Could you check a few things on this model? Use its own coordinates, in mm. A direction names the side the tool comes from. Give positions to 0.01 mm unless a question says otherwise; leave off trailing zeros. Write each loop counter-clockwise with the first axis right and the second up, starting at its lowest first coordinate (ties: lowest second). Pieces come first, ordered by that corner, then holes. Notation, with made-up numbers: M 49,-23 L 63,-23 A26 ccw 63,12 Z; hole C 78,-2.5 d1. An arc over 180 degrees is marked long. One line per item, written item: value.
```python
from build123d import *

# Parameters (mm, degrees)
BOSS_EXTRUDE1_DEPTH      = 7
BOSS_EXTRUDE2_DEPTH      = 1
SKETCH3_W                = 6.66403437
SKETCH3_H                = 33.73555596
CUT_EXTRUDE1_DEPTH       = 29.374724668
BOSS_EXTRUDE3_DEPTH      = 3.3
CUT_EXTRUDE2_DEPTH       = 3.7
SKETCH6_W                = 4
SKETCH6_H                = 16.6
CUT_EXTRUDE3_DEPTH       = 2.5
BOSS_EXTRUDE4_REACH      = 45.389
BOSS_EXTRUDE4_END_RADIUS = 19.25
SKETCH7_R                = 1.5


with BuildPart() as part:
    # Sketch1 → Boss-Extrude1 (new body)
    with BuildSketch(Plane(origin=(0, 0, 0), x_dir=(1, 0, 0), z_dir=(0, 1, 0))):
        with BuildLine():
            Line((-16, -10.703387314), (-16, 10.703387314))
            ThreePointArc((-16, 10.703387314), (19.25, 0), (-16, -10.703387314))
        make_face()
        with BuildLine():
            Line((-15, -10.395311443), (-15, 10.395311443))
            ThreePointArc((-15, 10.395311443), (18.25, 0), (-15, -10.395311443))
        make_face(mode=Mode.SUBTRACT)
    extrude(amount=BOSS_EXTRUDE1_DEPTH)

    # Sketch2 → Boss-Extrude2 (add)
    with BuildSketch(Plane.XZ):
        with BuildLine():
            Line((-16, 10.703387314), (-16, -10.703387314))
            ThreePointArc((-16, -10.703387314), (19.25, 0), (-16, 10.703387314))
        make_face()
    extrude(amount=BOSS_EXTRUDE2_DEPTH)

    # Sketch3 → Cut-Extrude1 (cut, through all)
    with BuildSketch(Plane(origin=(0, 7, 0), x_dir=(1, 0, 0), z_dir=(0, 1, 0))):
        with Locations((-18.332017185, -0.479198238)):
            Rectangle(SKETCH3_W, SKETCH3_H)
    extrude(amount=-CUT_EXTRUDE1_DEPTH, mode=Mode.SUBTRACT)

    # Sketch4 → Boss-Extrude3 (add)
    with BuildSketch(Plane(origin=(0, 0, 0), x_dir=(1, 0, 0), z_dir=(0, 1, 0))):
        Polygon((-15, 12.064928512), (-15, -12.064928512), (-13, -12.808688457), (-13, 12.808688457), align=None)
    extrude(amount=BOSS_EXTRUDE3_DEPTH)

    # Sketch5 → Cut-Extrude2 (cut)
    with BuildSketch(Plane(origin=(0, 7, 0), x_dir=(1, 0, 0), z_dir=(0, 1, 0))):
        Polygon((0, 0), (-15, -12.064928512), (-15, 12.064928512), align=None)
    extrude(amount=-CUT_EXTRUDE2_DEPTH, mode=Mode.SUBTRACT)

    # Sketch6 → Cut-Extrude3 (cut)
    with BuildSketch(Plane(origin=(0, 3.3, 0), x_dir=(1, 0, 0), z_dir=(0, 1, 0))):
        with Locations((-15, 0)):
            Rectangle(SKETCH6_W, SKETCH6_H)
    extrude(amount=-CUT_EXTRUDE3_DEPTH, mode=Mode.SUBTRACT)

    # Boss-Extrude4: up to this cylinder (the profile starts outside it)
    boss_extrude4_end = Plane(origin=(0, 0.5, 0), z_dir=(0, -1, 0)) * Cylinder(BOSS_EXTRUDE4_END_RADIUS, 130.278, mode=Mode.PRIVATE)
    # Sketch7 → Boss-Extrude4 (add, up to the surface)
    with BuildSketch(Plane.XY.offset(19), mode=Mode.PRIVATE) as boss_extrude4_sk1:
        with BuildLine():
            Line((-14, 2), (-14, -1))
            Line((-14, -1), (-6, -1))
            Line((-6, -1), (-6, 2))
            ThreePointArc((-6, 2), (-10, 6), (-14, 2))
        make_face()
        with Locations((-10, 2)):
            Circle(SKETCH7_R, mode=Mode.SUBTRACT)
    boss_extrude4_tool1 = extrude(boss_extrude4_sk1.sketch, amount=-BOSS_EXTRUDE4_REACH, mode=Mode.PRIVATE) - boss_extrude4_end
    boss_extrude4 = boss_extrude4_tool1.solids().sort_by_distance((-13.893699, 0.5, 19))[0]
    add(boss_extrude4)

    # Mirror1: Boss-Extrude4 across plane
    add(boss_extrude4.mirror(Plane.XY))


solid = part.part
```
1) If we section it at C-C, the plane y = 5.5: Write out the boundary of the cut face in (x, z), then the cut area to 3 significant figures.
Outcome:
outline: M -15,-12.06 A19.25 ccw -11.94,-15.1 L -11.94,-19 L -8.06,-19 L -8.06,-17.48 A19.25 ccw long -8.06,17.48 L -8.06,19 L -11.94,19 L -11.94,15.1 A19.25 ccw -15,12.06 L -14.22,11.44 A18.25 cw long -14.22,-11.44 Z
area: 113 mm^2
2) If we section it at A-A, the plane x = 0: Write out the boundary of the cut face in (y, z).
Outcome:
outline: M -1,-19.25 L 7,-19.25 L 7,-18.25 L 0,-18.25 L 0,18.25 L 7,18.25 L 7,19.25 L -1,19.25 Z
3) Please list where these lines run through material, in increasing order: L1, parallel to Z at x = 0, y = 3; L2, parallel to X at y = 2, z = -16.3; L3, parallel to X at y = 1, z = 16. Write a range as from..to.
Outcome:
L1: z = -19.25..-18.25, 18.25..19.25
L2: x = -14..-11.5, -10.24..-8.21, 8.21..10.24
L3: x = -14..-11.12, -10.7..-8.78, 8.78..10.7
4) If we section it at D-D, the plane x = -8: Write out the boundary of the cut face in (y, z), then the cut area to 3 significant figures.
Outcome:
outline: M -1,-19 L 5.46,-19 L 5.46,-17.51 L 7,-17.51 L 7,-16.4 L 0,-16.4 L 0,16.4 L 7,16.4 L 7,17.51 L 5.46,17.51 L 5.46,19 L -1,19 Z
area: 69.8 mm^2
5) We'd pull the mould along Z, two halves only. Please class faces 1 (the face through (-12, 3, 19)), 2 (the face through (19, 7, 0)), 3 (the face through (-14, 3.3, 10)): pulls with the +Z half, pulls with the -Z half, needs draft (parallel to the pull), parting line crosses it, or undercut.
Outcome:
face 1: pulls with the +Z half
face 2: needs draft
face 3: undercut
6) If we section it at B-B, the plane z = -6.5: Write out the boundary of the cut face in (x, y), then the cut area to 3 significant figures.
Outcome:
outline: M -15,-1 L 18.12,-1 L 18.12,7 L 17.05,7 L 17.05,0 L -13,0 L -13,0.8 L -15,0.8 Z
area: 42.2 mm^2
7) On a 3-axis mill with a long thin cutter (end or side, diameter ignored), from which of +Z, -Z, +X, -X, +Y, -Y can I reach the whole of each face in a straight line? I mean faces 4 (the face through (-14, 1, 16)), 5 (the face through (-14, 2, -8.3)), 6 (the face through (-13, 0.5, 0.2)). Say none if no direction works.
Outcome:
face 4: +Z, -X, +Y, -Y
face 5: -X, +Y
face 6: +Y
8) I'm going to push flat-ended pins straight in: pin 1 (2 mm diameter, centred on x = -3, y = 5, fed in from +Z); pin 2 (0.9 mm diameter, centred on y = 0, z = 15.5, fed in from -X); pin 3 (2 mm diameter, centred on x = -13.5, z = 10, fed in from +Y). Where does each tip first touch, or does it pass through?
Outcome:
pin 1: stops at z = 19.15
pin 2: stops at x = -14
pin 3: stops at y = 3.3
